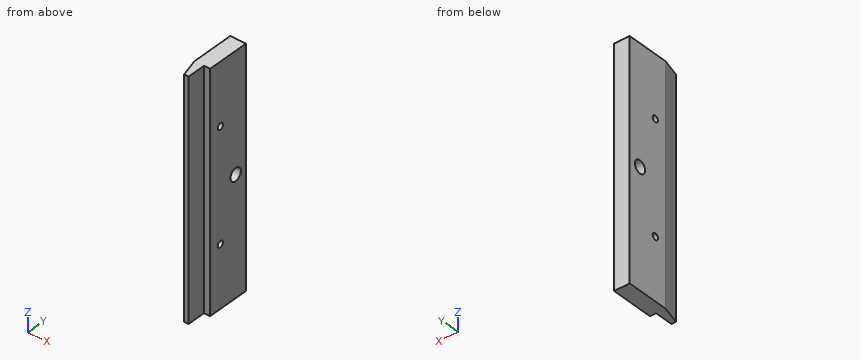
from build123d import *

# Parameters (mm, degrees)
SALIENTE_EXTRUIR1_DEPTH       = 95
TALADRO_ROSCADO_1_4_201_D     = 5.1054
TALADRO_DE_MARGEN_PARA_3_81_D = 10.0838


with BuildPart() as part:
    # Croquis1 → Saliente-Extruir1 (new, symmetric)
    with BuildSketch(Plane.XY):
        Polygon((6.35, -17.5), (1.35, -17.5), (1.35, -32.5), (-2.330762114, -32.5), (-6.35, -17.5), (-6.35, 17.5), (6.35, 17.5), align=None)
    extrude(amount=SALIENTE_EXTRUIR1_DEPTH, both=True)

    # Taladro roscado 1/4-201 (through all)
    with Locations(Plane(origin=(6.35, 0, 0), x_dir=(0, 0, -1), z_dir=(1, 0, 0))):
        with Locations((45.25, -7.5), (-45.25, -7.5)):
            Hole(TALADRO_ROSCADO_1_4_201_D / 2)

    # Taladro de margen para 3/81 (through all)
    with Locations(Plane(origin=(6.35, 0, 0), x_dir=(0, 0, -1), z_dir=(1, 0, 0))):
        with Locations((0, 7.5)):
            Hole(TALADRO_DE_MARGEN_PARA_3_81_D / 2)


solid = part.part
Geometry check sheet. Reference: the model listing, model coordinates, mm. Round coordinates to 2 decimals unless told otherwise and drop trailing zeros. Order: outer loops, then holes, each group sorted by start corner. A loop starts at its lowest first (then second) coordinate and runs counter-clockwise, first axis right, second up. Notation, with made-up numbers: (60.25, 65.25) -> (82.25, 65.25) arc R8 cw to (82.25, 71.25) -> close; hole circle Ø5 at (-14, -23.5). An arc over 180 degrees is marked (long way). Use one line per item in the form item = value.
1. Go/stop test with flat-tipped pins: pin 1 (3 mm diameter, centred on y = -24.5, z = 63, fed in from +X); pin 2 (2.5 mm diameter, centred on x = 5, z = 19, fed in from -Y); pin 3 (6 mm diameter, centred on y = -7.5, z = 45.25, fed in from +X); pin 4 (6 mm diameter, centred on y = 7.5, z = 0, fed in from +X). Record where each tip stops, or that it passes through.
Working result:
pin_1 = 1.35
pin_2 = -17.5
pin_3 = 6.35
pin_4 = through
2. Cross-section at C-C, the plane z = -11. Enter the section's corners in (x, y), plus the area to 3 significant figures.
Working result:
outline = (-6.35, -17.5) -> (-2.33, -32.5) -> (1.35, -32.5) -> (1.35, -17.5) -> (6.35, -17.5) -> (6.35, 17.5) -> (-6.35, 17.5) -> close
area = 530 mm^2
3. Scan lines: line 1 along Y through (x, z) = (1.5, 45.25); line 2 along Y through (x, z) = (-1, 45.25); line 3 along Z through (x, y) = (0.25, -7). Record each from-to range of solid material in increasing order. Write a range as from..to.
Working result:
line_1 = -17.5..-10.05, -4.95..17.5
line_2 = -32.5..-10.05, -4.95..17.5
line_3 = -95..-47.75, -42.75..42.75, 47.75..95
4. Cross-section at D-D, the plane x = -4.75. Enter the section's corners in (y, z).
Working result:
outline = (-23.47, -95) -> (17.5, -95) -> (17.5, 95) -> (-23.47, 95) -> close; hole circle Ø5.11 at (-7.5, -45.25); hole circle Ø5.11 at (-7.5, 45.25); hole circle Ø10.08 at (7.5, 0)
5. Cross-section at B-B, the plane y = 7.5. Enter the section's corners in (x, z), plus the area to 3 significant figures.
Working result:
outline = (-6.35, -95) -> (6.35, -95) -> (6.35, -5.04) -> (-6.35, -5.04) -> close; (-6.35, 5.04) -> (6.35, 5.04) -> (6.35, 95) -> (-6.35, 95) -> close
area = 2,280 mm^2
6. Cross-section at A-A, the plane z = 45.25. Enter the section's corners in (x, y), plus the area to 3 significant figures.
Working result:
outline = (-6.35, -17.5) -> (-2.33, -32.5) -> (1.35, -32.5) -> (1.35, -17.5) -> (6.35, -17.5) -> (6.35, -10.05) -> (-6.35, -10.05) -> close; (-6.35, -4.95) -> (6.35, -4.95) -> (6.35, 17.5) -> (-6.35, 17.5) -> close
area = 465 mm^2
